Can you work these out from the drawing? Everything is in mm from the part's minimum corner. Round coordinates to 2 decimals unless told otherwise and drop trailing zeros. Order: outer loops, then holes, each group sorted by start corner. A loop starts at its lowest first (then second) coordinate and runs counter-clockwise, first axis right, second up. Notation, with made-up numbers: (71, 52.5) -> (89, 52.5) arc R15 cw to (89, 63.5) -> close; hole circle Ø7 at (24, -5). An arc over 180 degrees is marked (long way). One line per item, written item: value.
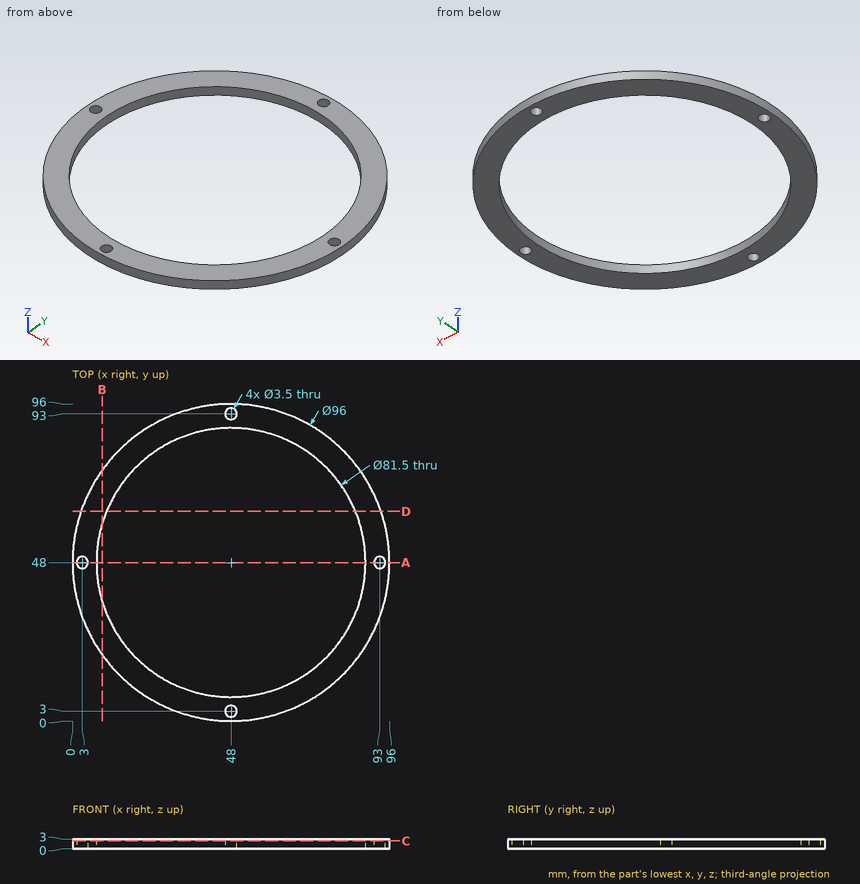
Q1. I want a section at B-B on x = 9. Write out the boundary of the cut face in (y, z), then the cut area to 3 significant figures.
Answers:
outline: (20.02, 0) -> (36.19, 0) -> (36.19, 3) -> (20.02, 3) -> close; (59.81, 0) -> (75.98, 0) -> (75.98, 3) -> (59.81, 3) -> close
area: 97.0 mm2
Q2. For P1, Ø1.5, axis at y = 70.5, z = 0.5, coming from the +X side; P2, Ø4, axis at x = 3, y = 48, coming from the -Z side, each with a flat end and sliding along its axis, tell me the tip position at first contact or that it passes through.
Answers:
P1: x = 90.79
P2: z = 0
Q3. I want a section at C-C on z = 2.4. Write out the boundary of the cut face in (x, y).
Answers:
outline: circle Ø96 at (48, 48); hole circle Ø3.5 at (3, 48); hole circle Ø81.5 at (48, 48); hole circle Ø3.5 at (48, 3); hole circle Ø3.5 at (48, 93); hole circle Ø3.5 at (93, 48)
Q4. I want a section at A-A on y = 48. Write out the boundary of the cut face in (x, z), then the cut area to 3 significant figures.
Answers:
outline: (0, 0) -> (1.25, 0) -> (1.25, 3) -> (0, 3) -> close; (4.75, 0) -> (7.25, 0) -> (7.25, 3) -> (4.75, 3) -> close; (88.75, 0) -> (91.25, 0) -> (91.25, 3) -> (88.75, 3) -> close; (94.75, 0) -> (96, 0) -> (96, 3) -> (94.75, 3) -> close
area: 22.5 mm2
Q5. I want a section at D-D on y = 63.5. Write out the boundary of the cut face in (x, z).
Answers:
outline: (2.57, 0) -> (10.31, 0) -> (10.31, 3) -> (2.57, 3) -> close; (85.69, 0) -> (93.43, 0) -> (93.43, 3) -> (85.69, 3) -> close
Q6. I need wall thicknesses on line 1 along Y through (x, z) = (48, 1.2); line 2 along X through (y, z) = (42, 1.9); line 3 along X through (y, z) = (32.5, 1.65). Which ranges of each line are inside material? Lowest first, please.
Answers:
line 1: 0 to 1.25, 4.75 to 7.25, 88.75 to 91.25, 94.75 to 96
line 2: 0.38 to 7.69, 88.31 to 95.62
line 3: 2.57 to 10.31, 85.69 to 93.43
